```python
from build123d import *

# Parameters (mm, degrees)
CUT_EXTRUDE1_DEPTH  = 5
CUT_EXTRUDE3_DEPTH  = 45
SKETCH8_R           = 40
CUT_EXTRUDE4_DEPTH  = 32
FILLET1_R           = 7
FILLET2_R           = 7
CUT_REVOLVE1_START  = 17
CUT_REVOLVE1_DEPTH  = 30.5
CUT_EXTRUDE12_DEPTH = 5
SKETCH18_W          = 13
SKETCH18_H          = 8
CUT_EXTRUDE13_DEPTH = 5
SKETCH20_W          = 84
SKETCH20_H          = 7
CUT_EXTRUDE15_DEPTH = 5
SKETCH19_R          = 1.35
CUT_EXTRUDE14_DEPTH = 8


# Read off the part's stored shape, not the designer's step: Cut-Revolve1
with BuildPart() as part:
    # Sketch1 → Revolve1 (revolve)
    with BuildSketch(Plane.XY, mode=Mode.PRIVATE) as revolve1_sk:
        with BuildLine():
            Line((22.5, 0), (23, 0))
            ThreePointArc((23, 0), (24.414213562, 0.585786438), (25, 2))
            Line((25, 2), (25, 13))
            Line((25, 13), (40, 13))
            ThreePointArc((40, 13), (41.414213562, 13.585786438), (42, 15))
            Line((42, 15), (42, 50))
            ThreePointArc((42, 50), (40.535533906, 53.535533906), (37, 55))
            Line((37, 55), (0, 55))
            Line((0, 55), (0, 13))
            Line((0, 13), (22.5, 13))
            Line((22.5, 13), (22.5, 0))
        make_face()
    revolve(revolve1_sk.sketch.rotate(Axis((0, 2, 0), (0, 1, 0)), 90), axis=Axis((0, 2, 0), (0, 1, 0)))

    # Sketch5 → Cut-Extrude1 (cut)
    with BuildSketch(Plane(origin=(0, 55, 0), x_dir=(1, 0, 0), z_dir=(0, 1, 0))):
        with BuildLine():
            Line((-42, 0), (-40, 0))
            Line((-40, 0), (40, 0))
            Line((40, 0), (42, 0))
            ThreePointArc((42, 0), (0, 42), (-42, 0))
        make_face()
    extrude(amount=-CUT_EXTRUDE1_DEPTH, mode=Mode.SUBTRACT)

    # Sketch7 → Cut-Extrude3 (cut)
    with BuildSketch(Plane.XZ.offset(-13)):
        with BuildLine():
            Line((-21, 0), (21, 0))
            ThreePointArc((21, 0), (0, -21), (-21, 0))
        make_face()
    extrude(amount=-CUT_EXTRUDE3_DEPTH, mode=Mode.SUBTRACT)

    # Sketch8 → Cut-Extrude4 (cut)
    with BuildSketch(Plane(origin=(0, 47.5, 0), x_dir=(1, 0, 0), z_dir=(0, 1, 0))):
        with Locations(Location((0, 0, 0), (0, 0, 270))):
            Circle(SKETCH8_R)
        with BuildLine():
            Line((22.912878475, -2), (-22.912878475, -2))
            ThreePointArc((-22.912878475, -2), (0, 23), (22.912878475, -2))
        make_face(mode=Mode.SUBTRACT)
    extrude(amount=-CUT_EXTRUDE4_DEPTH, mode=Mode.SUBTRACT)

    # Fillet1
    fillet1_edges = [part.edges().sort_by_distance(p)[0] for p in [
        (21, 31.5, 0),
        (-21, 31.5, 0),
    ]]
    fillet(fillet1_edges, radius=FILLET1_R)

    # Fillet2
    fillet2_edges = [part.edges().sort_by_distance(p)[0] for p in [
        (-22.912878475, 31.5, 2),
        (22.912878475, 31.5, 2),
    ]]
    fillet(fillet2_edges, radius=FILLET2_R)

    # Cut-Revolve1 outline → Cut-Revolve1 (cut)
    with BuildSketch(Plane(origin=(0, 0, 0), x_dir=(1, 0, 0), z_dir=(0, 1, 0)).offset(CUT_REVOLVE1_START)):
        with BuildLine():
            Line((-34.641016151, -20), (-36.373066959, -21))
            ThreePointArc((-36.373066959, -21), (0, -42), (36.373066959, -21))
            Line((36.373066959, -21), (34.641016151, -20))
            ThreePointArc((34.641016151, -20), (0, -40), (-34.641016151, -20))
        make_face()
    extrude(amount=CUT_REVOLVE1_DEPTH, mode=Mode.SUBTRACT)

    # Sketch15 → Cut-Extrude12 (cut)
    with BuildSketch(Plane(origin=(0, 15.5, 0), x_dir=(1, 0, 0), z_dir=(0, 1, 0))):
        with BuildLine():
            Line((-28.124355653, -3.514579578), (-26.124355653, -3.514579578))
            ThreePointArc((-26.124355653, -3.514579578), (-24.710142091, -2.928793141), (-24.124355653, -1.514579578))
            Line((-24.124355653, -1.514579578), (-24.124355653, 8.485420422))
            ThreePointArc((-24.124355653, 8.485420422), (-24.710142091, 9.899633984), (-26.124355653, 10.485420422))
            Line((-26.124355653, 10.485420422), (-28.124355653, 10.485420422))
            ThreePointArc((-28.124355653, 10.485420422), (-29.538569215, 9.899633984), (-30.124355653, 8.485420422))
            Line((-30.124355653, 8.485420422), (-30.124355653, -1.514579578))
            ThreePointArc((-30.124355653, -1.514579578), (-29.538569215, -2.928793141), (-28.124355653, -3.514579578))
        make_face()
    extrude(amount=-CUT_EXTRUDE12_DEPTH, mode=Mode.SUBTRACT)

    # Sketch18 → Cut-Extrude13 (cut)
    with BuildSketch(Plane(origin=(0, 50, 0), x_dir=(1, 0, 0), z_dir=(0, 1, 0))):
        with Locations((0.796512215, 32.951769165)):
            Rectangle(SKETCH18_W, SKETCH18_H)
    extrude(amount=-CUT_EXTRUDE13_DEPTH, mode=Mode.SUBTRACT)

    # Sketch20 → Cut-Extrude15 (cut)
    with BuildSketch(Plane(origin=(0, 55, 0), x_dir=(1, 0, 0), z_dir=(0, 1, 0))):
        with Locations((0, -3.5)):
            Rectangle(SKETCH20_W, SKETCH20_H)
    extrude(amount=-CUT_EXTRUDE15_DEPTH, mode=Mode.SUBTRACT)

    # Sketch19 → Cut-Extrude14 (cut)
    with BuildSketch(Plane(origin=(0, 0, 7), x_dir=(-1, 0, 0), z_dir=(0, 0, -1))):
        with Locations((0, 52.5)):
            Circle(SKETCH19_R)
        with Locations((-29.412558482, 52.5)):
            Circle(SKETCH19_R)
        with Locations((29.412558482, 52.5)):
            Circle(SKETCH19_R)
    extrude(amount=-CUT_EXTRUDE14_DEPTH, mode=Mode.SUBTRACT)


solid = part.part
```
Geometry: final body of the model. Coordinates: model frame, mm. A direction names the side the tool comes from. Give positions to 0.01 mm unless a question says otherwise; leave off trailing zeros. Loops run counter-clockwise (first coordinate to the right, second up) from the corner with the lowest first, then second, coordinate; pieces in that order, holes last. Notation, with made-up numbers: (66, -31.5) -> (105, -31.5) arc R21 cw to (105, -0.5) -> close; hole circle Ø9 at (17, -2.75). An arc over 180 degrees is marked (long way). Use CSV: the item, a comma, the result in double quotes.
(1) Access query for faces 1 (the face through (-7.509, 7.577, -23.846)), 2 (the face through (1, 15.5, 8)), 3 (the face through (-5.703, 49, -33)), 4 (the face through (29, 53, 15)). Directions: +Z, -Z, +X, -X, +Y, -Y. A direction counts if a zero-diameter tool reaches every point of the face in a straight line with its end or side. Return the directions, or none.
From the geometry:
face 1,"-Y"
face 2,"none"
face 3,"+Y"
face 4,"-Z"
(2) First-contact query: P1, Ø12, axis at x = -19, y = 13.5, coming from the -Z side; P2, Ø1.5, axis at y = 12, z = -5, coming from the -X side; P3, Ø1.5, axis at x = -21.5, z = -15, coming from the +Y side. Flat tips, straight axial feed; report the tip coordinate or a pass-through.
From the geometry:
P1,"z = -39.88"
P2,"x = -24.12"
P3,"y = 50"
(3) Cut plane A-A (y = 31.5). Output: boundary loops of the cut face in (x, z), plus the area to 3 significant figures.
From the geometry:
outline,"(-36.37, 21) arc R42 ccw (long way) to (36.37, 21) -> (34.64, 20) arc R40 cw (long way) to (-34.64, 20) -> close; (-21.85, -7.19) arc R23 ccw to (21.85, -7.19) arc R7 ccw to (15.2, 2) -> (-15.2, 2) arc R7 ccw to start; hole (-18.19, -10.5) arc R21 ccw to (18.19, -10.5) arc R7 ccw to (12.12, 0) -> (-12.12, 0) arc R7 ccw to start"
area,"586 mm^2"
(4) Cut plane D-D (y = 52.5). Output: boundary loops of the cut face in (x, z).
From the geometry:
outline,"(-40.73, 7) -> (-30.76, 7) -> (-30.76, 15) -> (-28.06, 15) -> (-28.06, 7) -> (-1.35, 7) -> (-1.35, 15) -> (1.35, 15) -> (1.35, 7) -> (28.06, 7) -> (28.06, 15) -> (30.76, 15) -> (30.76, 7) -> (40.73, 7) arc R41.33 ccw to start"
(5) Cut plane B-B (z = -15). Count the separate pieces of the cut face and the enclosed holes in it, plus the area to 3 significant figures.
From the geometry:
separate pieces,"2"
enclosed holes,"2"
area,"638 mm^2"
(6) Ray query, line 1 along Y through (x, z) = (-14.5, 22.5); line 2 along Y through (x, z) = (-22, -19.5); line 3 along X through (y, z) = (8, 0). Return the intervals inside material, ascending. Write a range as [from, to].
From the geometry:
line 1,"[13, 15.5], [47.5, 55]"
line 2,"[13, 15.5], [47.5, 50]"
line 3,"[-25, -22.5], [22.5, 25]"
(7) Pull-direction query (Z, two-part tool) for faces 5 (the face through (0, 17, 41)), 6 (the face through (-24, 32, -32)), 7 (the face through (-29, 53, 15)); classes: released by +Z, released by -Z, zero draft, split by the parting line, or undercut.
From the geometry:
face 5,"zero draft"
face 6,"undercut"
face 7,"released by -Z"
